Here's how the part is built. I have some questions about the finished solid (model axes, mm). Face numbers are marked on the shaded views. A direction names the side the tool comes from. Coordinates: 2 decimals unless noted, no trailing zeros. Order: outer loops, then holes, each group sorted by start corner. A loop starts at its lowest first (then second) coordinate and runs counter-clockwise, first axis right, second up. Notation, with made-up numbers: (78, 5) - (97, 5) arc R37 cw to (97, 44) - close; hole circle Ø9 at (79.25, 23.25). An arc over 180 degrees is marked (long way). Answer as CSV lines item,"result". Start each with the question number.
Q1. For pin 1 Ø1 at (y, z) = (4.5, 105.5) entering from +X; pin 2 Ø5 at (x, y) = (38.3, -0.36) entering from -Z; pin 3 Ø12 at (x, z) = (-22.5, 51) entering from +Y; pin 4 Ø3.5 at (x, z) = (-5.5, 5.5) entering from -Y, each with a flat end and sliding along its axis, tell me the tip position at first contact or that it passes through.
Q2. I need wall thicknesses on line 1 (Y direction, x = -0.5, z = 128); line 2 (X direction, y = -1.5, z = 102); line 3 (X direction, y = -2.5, z = 110). Which ranges of each line are inside material? Lowest first, please.
Q3. Suppose I cut it at A-A (x = 22). Please give me the cut outline in (y, z) (3 decimals).
Q4. Suppose I cut it at B-B (y = 1). Please give me the cut outline in (x, z).
Q5. For the marked faces 1, 2 and 3, which set-ups out of +Z, -Z, +X, -X, +Y, -Y let a thin tool reach every point of the face, with its end or its side?
Q6. Suppose I cut it at C-C (z = 109). Please give me the cut outline in (x, y) (3 decimals).
from build123d import *

# Parameters (mm, degrees)
SKETCH1_R           = 3.175
BOSS_EXTRUDE1_DEPTH = 146.05
BOSS_EXTRUDE2_DEPTH = 3.175
SKETCH3_W           = 58.42
SKETCH3_H           = 9.525
BOSS_EXTRUDE3_DEPTH = 3.175
BOSS_EXTRUDE4_DEPTH = 146.05
CUT_EXTRUDE1_DEPTH  = 146.05


with BuildPart() as part:
    # Sketch1 → Boss-Extrude1 (new body)
    with BuildSketch(Plane.XY):
        with BuildLine():
            Line((-33.243254954, 2.815203929), (-25.623254954, -3.534796071))
            Line((-25.623254954, -3.534796071), (32.796745046, -3.534796071))
            ThreePointArc((32.796745046, -3.534796071), (44.64600636, -0.359796071), (32.796745046, 2.815203929))
            Line((32.796745046, 2.815203929), (-33.243254954, 2.815203929))
        make_face()
        with Locations((38.29600636, -0.359796071)):
            Circle(SKETCH1_R, mode=Mode.SUBTRACT)
    extrude(amount=BOSS_EXTRUDE1_DEPTH)

    # Sketch2 → Boss-Extrude2 (add)
    with BuildSketch(Plane.XY.offset(3.175)):
        Polygon((-22.448254954, 2.815203929), (-25.623254954, 2.815203929), (-25.623254954, 12.340203929), (32.796745046, 12.340203929), (32.796745046, 2.815203929), (29.621745046, 2.815203929), (29.621745046, 9.165203929), (-22.448254954, 9.165203929), align=None)
    extrude(amount=BOSS_EXTRUDE2_DEPTH)

    # Sketch3 → Boss-Extrude3 (add)
    with BuildSketch(Plane.XY.offset(6.35)):
        with Locations((3.586745046, 7.577703929)):
            Rectangle(SKETCH3_W, SKETCH3_H)
    extrude(amount=BOSS_EXTRUDE3_DEPTH)

    # Sketch4 → Boss-Extrude4 (add)
    with BuildSketch(Plane.XY.offset(146.05)):
        Polygon((-33.243254954, 2.815203929), (-33.243254954, -3.534796071), (-25.623254954, -3.534796071), align=None)
    extrude(amount=-BOSS_EXTRUDE4_DEPTH)

    # Sketch5 → Cut-Extrude1 (cut)
    with BuildSketch(Plane.XY.offset(146.05)):
        Polygon((-33.243254954, -3.534796071), (-25.623254954, 2.815203929), (-33.243254954, 2.815203929), align=None)
    extrude(amount=-CUT_EXTRUDE1_DEPTH, mode=Mode.SUBTRACT)


solid = part.part
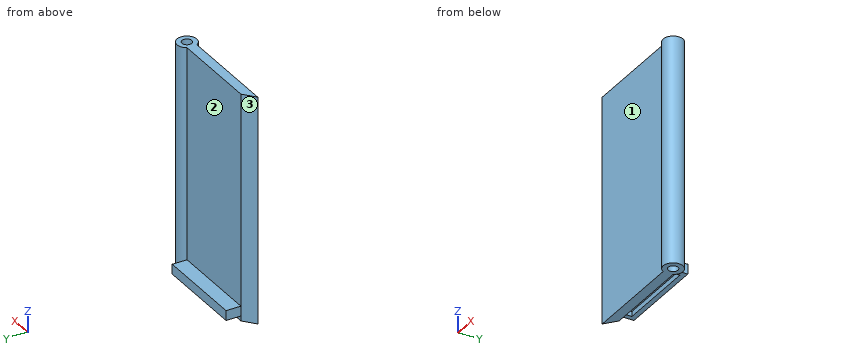
Here are the results:
1,pin 1,"stops at x = 42.91"
1,pin 2,"passes through"
1,pin 3,"stops at y = 2.82"
1,pin 4,"stops at y = -3.53"
2,line 1,"y = -3.53 to 2.82"
2,line 2,"x = -30.8 to 35.33, 41.26 to 44.54"
2,line 3,"x = -32 to 35.95, 40.64 to 44.27"
3,outline,"(-3.535, 0) - (2.815, 0) - (2.815, 6.35) - (9.165, 6.35) - (9.165, 3.175) - (12.34, 3.175) - (12.34, 9.525) - (2.815, 9.525) - (2.815, 146.05) - (-3.535, 146.05) - close"
4,outline,"(-27.8, 0) - (35.43, 0) - (35.43, 146.05) - (-27.8, 146.05) - close; (41.17, 0) - (44.5, 0) - (44.5, 146.05) - (41.17, 146.05) - close"
5,face 1,"+Z, -Z, -X, -Y"
5,face 2,"+Z, -X, +Y"
5,face 3,"+Z, -Z, -X, +Y"
6,outline,"(-33.243, -3.535) - (32.797, -3.535) arc R6.35 ccw (long way) to (32.797, 2.815) - (-25.623, 2.815) - close; hole circle Ø6.35 at (38.296, -0.36)"
